Work out the finished part from the listing and answer in its coordinate system (mm). Coordinates: 2 decimals unless noted, no trailing zeros. Loops run counter-clockwise (first coordinate to the right, second up) from the corner with the lowest first, then second, coordinate; pieces in that order, holes last.
```python
from build123d import *

# Parameters (mm, degrees)
F1_DEPTH      = 12.7
F1_DEPTH_BACK = 12.7
F2_W          = 10.16
F2_H          = 10.16
F3_DEPTH      = 3.175
F5_DEPTH      = 3.175
F6_R          = 1.27
F7_R          = 4.445
F8_D          = 10.16
F8_DEPTH      = 3.175
F8_TIP        = 3.0523719447


with BuildPart() as f1:
    # F0 (on Front) → F1 (new body, two sides)
    with BuildSketch(Plane.XZ) as f1_sk:
        Polygon((3.175, 0), (-3.175, 0), (-4.5684314445, 53.213), (-7.7423434513, 53.1298881891), (-6.2679480652, -3.175), (6.2679480652, -3.175), (7.7423434513, 53.1298881891), (4.5684314445, 53.213), align=None)
    extrude(amount=F1_DEPTH)
    extrude(f1_sk.sketch, amount=-F1_DEPTH_BACK)

    # F2 (on face) → F3 (cut, through all)
    with BuildSketch(Plane(origin=(6.3467363932, 0, -0.1661951414), x_dir=(0, 1, 0), z_dir=(0.999657325, 0, -0.0261769483))):
        with BuildLine():
            ThreePointArc((-12.7, 40.6143528277), (-8.9802561276, 49.5946089422), (-1.86e-08, 53.3143528277))
            Line((-1.86e-08, 53.3143528277), (-12.7, 53.3143528277))
            Line((-12.7, 53.3143528277), (-12.7, 40.6143528277))
        make_face()
        with BuildLine():
            ThreePointArc((-1.86e-08, 53.3143528277), (8.9802561145, 49.5946089553), (12.7, 40.6143528277))
            Line((12.7, 40.6143528277), (12.7, 53.3143528277))
            Line((12.7, 53.3143528277), (-1.86e-08, 53.3143528277))
        make_face()
        with Locations((0, 40.6143528277)):
            Rectangle(F2_W, F2_H)
    extrude(amount=-F3_DEPTH, mode=Mode.SUBTRACT)

    # F4 (on face) → F5 (cut, through all)
    with BuildSketch(Plane(origin=(-6.3467363932, 0, -0.1661951414), x_dir=(0, -1, 0), z_dir=(-0.999657325, 0, -0.0261769483))):
        with BuildLine():
            ThreePointArc((-12.7, 40.6143528277), (-8.9802561029, 49.594608967), (5.15e-08, 53.3143528277))
            Line((5.15e-08, 53.3143528277), (-12.7, 53.3143528277))
            Line((-12.7, 53.3143528277), (-12.7, 40.6143528277))
        make_face()
        with BuildLine():
            ThreePointArc((5.15e-08, 53.3143528277), (8.9802561393, 49.5946089305), (12.7, 40.6143528277))
            Line((12.7, 40.6143528277), (12.7, 53.3143528277))
            Line((12.7, 53.3143528277), (5.15e-08, 53.3143528277))
        make_face()
    extrude(amount=-F5_DEPTH, mode=Mode.SUBTRACT)

    # F6
    f6_edges = [f1.edges().sort_by_distance(p)[0] for p in [
        (3.175, 0, 0),
        (-3.175, 0, 0),
    ]]
    fillet(f6_edges, radius=F6_R)

    # F7
    f7_edges = [f1.edges().sort_by_distance(p)[0] for p in [
        (6.267948, 0, -3.175),
        (-6.267948, 0, -3.175),
    ]]
    fillet(f7_edges, radius=F7_R)

    # F8
    with Locations(Plane(origin=(-6.3467363932, 0, -0.1661951414), x_dir=(0, -1, 0), z_dir=(-0.999657325, 0, -0.0261769483))):
        with Locations((0, 40.6143528277)):
            Hole(F8_D / 2, depth=F8_DEPTH)
            with Locations((0, 0, -(F8_DEPTH + F8_TIP / 2))):  # 118° drill point
                Cone(0, F8_D / 2, F8_TIP, mode=Mode.SUBTRACT)


solid = f1.part
```
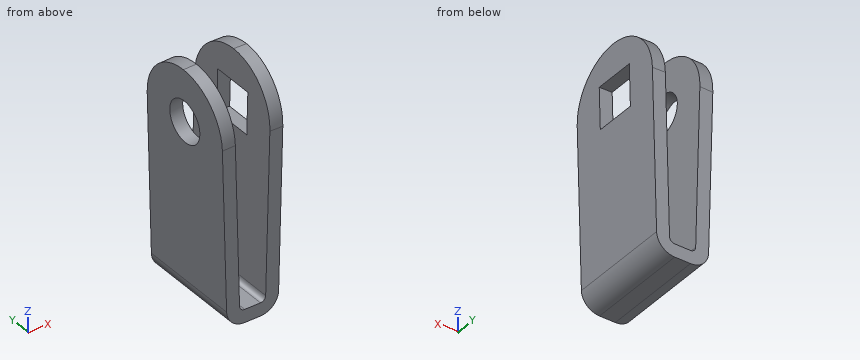
1. Straight lines are drawn through the part: probe 1 along Z at (x, y) = (-1.5, -10) (3 decimals); probe 2 along X at (y, z) = (2.75, 48); probe 3 along X at (y, z) = (-10.5, 11.5). For each, find the intervals that lie inside material, in ascending order.
2. A cutting plane is placed at B-B, the plane y = -2.25. Give the vertices of the cut face in (x, z) (1 decimal).
3. A cutting plane is placed at A-A, the plane z = 23. Give the vertices of the cut face in (x, y).
4. A cutting plane is placed at C-C, the plane y = -10.25. Give the vertices of the cut face in (x, z) (3 decimals), then the cut area to 3 significant figures.
5. A cutting plane is placed at D-D, the plane x = -0.5. Give the vertices of the cut face in (y, z) (3 decimals), then the cut area to 3 significant figures.
6. Each of these flat-tipped pins is pushed along its axis until it touches: P1, Ø1.5, axis at x = -4, y = -3, coming from the +Z side; P2, Ø5, axis at y = 8, z = 43.5, coming from the +X side; P3, Ø3, axis at y = -8, z = 27, coming from the +X side. Where does it stop, or does it pass through?
Answers below:
1. probe 1: z = -3.175 to 0
1. probe 2: x = -7.61 to -4.43, 4.43 to 7.61
1. probe 3: x = -6.65 to -3.48, 3.48 to 6.65
2. outline: (-7.7, 52.9) - (-7.5, 45) - (-4.4, 45.1) - (-4.6, 53) - close; (-7.3, 35.9) - (-6.4, 1.2) arc R4.4 ccw to (-1.9, -3.2) - (1.9, -3.2) arc R4.4 ccw to (6.4, 1.2) - (7.3, 35.4) - (4.1, 35.4) - (3.2, 1.2) arc R1.3 cw to (1.9, 0) - (-1.9, 0) arc R1.3 cw to (-3.2, 1.2) - (-4.1, 36) - close; (4.4, 45.6) - (7.5, 45.5) - (7.7, 52.9) - (4.6, 53) - close
3. outline: (-6.95, -12.7) - (-3.78, -12.7) - (-3.78, 12.7) - (-6.95, 12.7) - close; (3.78, -12.7) - (6.95, -12.7) - (6.95, 12.7) - (3.78, 12.7) - close
4. outline: (-7.606, 47.93) - (-6.381, 1.154) arc R4.445 ccw to (-1.938, -3.175) - (1.938, -3.175) arc R4.445 ccw to (6.381, 1.154) - (7.606, 47.93) - (4.432, 48.013) - (3.207, 1.237) arc R1.27 cw to (1.938, 0) - (-1.938, 0) arc R1.27 cw to (-3.207, 1.237) - (-4.432, 48.013) - close
4. area: 337 mm2
5. outline: (-12.7, -3.175) - (12.7, -3.175) - (12.7, 0) - (-12.7, 0) - close
5. area: 80.6 mm2
6. P1: stops at z = 52.96
6. P2: stops at x = 7.56
6. P3: stops at x = 7.1
